Read the model definition and answer for the solid it produces. Units are mm, in the model's axes. Face numbers are marked on the shaded views. A direction names the side the tool comes from. Round coordinates to 2 decimals unless told otherwise and drop trailing zeros. Order: outer loops, then holes, each group sorted by start corner. A loop starts at its lowest first (then second) coordinate and runs counter-clockwise, first axis right, second up. Notation, with made-up numbers: (4, -1.75) - (16, -1.75) arc R11 ccw to (16, 4.25) - close; hole circle Ø9 at (3.25, 26.5). An arc over 180 degrees is marked (long way). Put each result on its own line as item: value. Start each with the question number.
Q1. Section D-D on x = 36.5 is taken. Give the vertices of the cut face in (y, z), then the cut area to 3 significant figures.
Q2. Each of these flat-tipped pins is pushed along its axis until it touches: pin 1 Ø3.5 at (y, z) = (-22, -43.5) entering from -X; pin 2 Ø2 at (y, z) = (-4.5, 16.5) entering from -X; pin 3 Ø1 at (y, z) = (-8.5, -27.5) entering from -X. Where does it stop, or does it pass through?
Q3. Which of the six approach directions +Z, -Z, +X, -X, +Y, -Y give full straight-line access (tool end or side, diameter ignored) to the marked faces 5, 6, 7, 8 and 9?
Q4. For a pull along X with two mould halves and no side action, classify the marked faces 1, 2, 3 and 4 as pulls with the +X half, pulls with the -X half, needs draft (parallel to the pull), parting line crosses it, or undercut.
Q5. Section C-C on y = -19.5 is taken. Give the vertices of the cut face in (x, z) (3 decimals).
Q6. Section A-A on x = 20 is taken. Give the vertices of the cut face in (y, z), then the cut area to 3 significant figures.
Q7. Find the intervals of material crossed by line 1 along Z through (x, y) = (-2, -20.25); line 2 along Z through (x, y) = (49, -11.5); line 3 along Z through (x, y) = (-1, -26), in increasing order. Write a range as from..to.
Q8. Section B-B on z = -23.5 is taken. Give the vertices of the cut face in (x, y), then the cut area to 3 significant figures.
from build123d import *

# Parameters (mm, degrees)
F0_W      = 71.12
F0_H      = 28.448
F1_DEPTH  = 28.448
F3_DEPTH  = 25.4
F4_DEPTH  = 25.4
F6_DEPTH  = 29.3733245078
F8_DEPTH  = 29.3562148671
F9_W      = 26.5992027439
F9_H      = 25.4
F10_DEPTH = 29.3562148671
F12_DEPTH = 50.8
F14_DEPTH = 25.3715035059
F16_DEPTH = 29.4182237139
F18_DEPTH = 29.4182237139


with BuildPart() as f1:
    # F0 (on Front) → F1 (new body)
    with BuildSketch(Plane.XZ):
        with Locations((4.2755420916, -14.224)):
            Rectangle(F0_W, F0_H)
    extrude(amount=F1_DEPTH)

    # F2 (on face) → F3 (join)
    with BuildSketch(Plane.XY):
        Polygon((39.8355420916, -6.35), (-31.2844579084, -6.35), (-31.2844579084, -21.59), (-24.3643354625, -21.59), (-24.3643354625, -26.416), (39.8355420916, -26.416), align=None)
        Polygon((39.8355420916, 0), (39.8355420916, -6.35), (39.8355420916, -26.416), (39.8355420916, -28.448), (66.4746039532, -29.3723245078), (66.4906352758, 0), align=None)
    extrude(amount=-F3_DEPTH)

    # F2 (on face) → F4 (join)
    with BuildSketch(Plane.XY):
        Polygon((39.8355420916, -6.35), (-31.2844579084, -6.35), (-31.2844579084, -21.59), (-24.3643354625, -21.59), (-24.3643354625, -26.416), (39.8355420916, -26.416), (39.8355420916, -28.448), (66.4746039532, -29.3723245078), (66.4906352758, 0), (39.8355420916, 0), align=None)
    extrude(amount=F4_DEPTH)

    # F5 (on Front) → F6 (cut, through all)
    with BuildSketch(Plane.XZ):
        with BuildLine():
            Line((13.9288037957, 18.2963101068), (-12.0401520726, 18.2963101068))
            ThreePointArc((-12.0401520726, 18.2963101068), (-16.6437398491, 13.6927223303), (-12.0401520726, 9.0891345539))
            Line((-12.0401520726, 9.0891345539), (13.9288037957, 9.0891345539))
            ThreePointArc((13.9288037957, 9.0891345539), (18.5323915722, 13.6927223303), (13.9288037957, 18.2963101068))
        make_face()
        Polygon((69.9178975219, 28.448), (39.8913989174, 0), (69.9178975219, 0), align=None)
    extrude(amount=F6_DEPTH, mode=Mode.SUBTRACT)

    # F7 (on face) → F8 (cut, through all)
    with BuildSketch(Plane(origin=(-0.9380015967, -27.0332360006, 0), x_dir=(0.9993985644, -0.0346772191, 0), z_dir=(-0.0346772191, -0.9993985644, 0))):
        Polygon((54.266725333, 12.7), (40.7980811078, 12.7), (40.8539715481, 0), align=None)
    extrude(amount=-F8_DEPTH, mode=Mode.SUBTRACT)

    # F9 (on face) → F10 (cut, through all)
    with BuildSketch(Plane(origin=(-0.9380015967, -27.0332360006, 0), x_dir=(0.9993985644, -0.0346772191, 0), z_dir=(-0.0346772191, -0.9993985644, 0))):
        with Locations((54.15357292, -12.7)):
            Rectangle(F9_W, F9_H)
    extrude(amount=-F10_DEPTH, mode=Mode.SUBTRACT)

    # F11 (on Top) → F12 (join)
    with BuildSketch(Plane.XY):
        Polygon((39.5289533985, -6.35), (-31.5910466015, -6.35), (-31.0273190044, -20.828), (-20.2347878367, -20.828), (-20.2347878367, -25.3705035059), (33.4493406117, -25.3705035059), (39.5289533985, -25.3705035059), (39.5289533985, -28.8873665619), (65.7633790028, -29.4085801184), (65.7633790028, 0), (39.5289533985, 0), align=None)
    extrude(amount=-F12_DEPTH)

    # F13 (on face) → F14 (cut, through all)
    with BuildSketch(Plane.XZ.offset(25.3705035059)):
        with BuildLine():
            Line((18.4132819485, -33.5730523437), (-10.3250071326, -33.5730523437))
            ThreePointArc((-10.3250071326, -33.5730523437), (-14.1350071326, -37.3830523437), (-10.3250071326, -41.1930523437))
            Line((-10.3250071326, -41.1930523437), (18.4132819485, -41.1930523437))
            ThreePointArc((18.4132819485, -41.1930523437), (22.4639207193, -37.3830523437), (18.4132819485, -33.5730523437))
        make_face()
    extrude(amount=-F14_DEPTH, mode=Mode.SUBTRACT)

    # F15 (on face) → F16 (cut, through all)
    with BuildSketch(Plane(origin=(-0.5580978428, -28.0909353817, 0), x_dir=(0.9998026988, -0.0198636223, 0), z_dir=(-0.0198636223, -0.9998026988, 0))):
        Polygon((66.3345647354, 0), (40.0949620257, 0), (40.0949620257, -29.1759762913), (66.3345647354, -50.8), align=None)
    extrude(amount=-F16_DEPTH, mode=Mode.SUBTRACT)

    # F17 (on face) → F18 (cut, through all)
    with BuildSketch(Plane(origin=(-0.5580978428, -28.0909353817, 0), x_dir=(0.9998026988, -0.0198636223, 0), z_dir=(-0.0198636223, -0.9998026988, 0))):
        Polygon((50.5786476823, -37.8155685024), (40.0949620257, -29.1759762913), (40.0949620257, -37.8155685024), align=None)
    extrude(amount=-F18_DEPTH, mode=Mode.SUBTRACT)


solid = f1.part
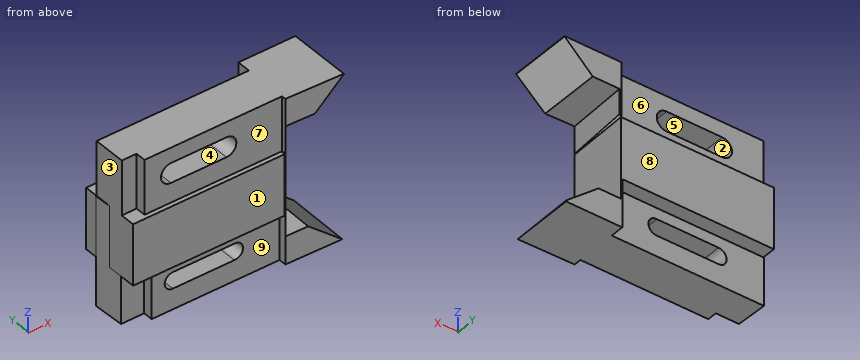
Findings:
1. outline: (-28.45, -28.45) - (-25.37, -28.45) - (-25.37, -50.8) - (-6.35, -50.8) - (-6.35, -28.45) - (0, -28.45) - (0, 0) - (-6.35, 0) - (-6.35, 25.4) - (-26.42, 25.4) - (-26.42, 0) - (-28.45, 0) - close
1. area: 1,740 mm2
2. pin 1: x = -31.05
2. pin 2: x = 39.84
2. pin 3: x = -31.53
3. face 5: +Y, -Y
3. face 6: +Z, -X, +Y
3. face 7: +Z, -X, -Y
3. face 8: +Z, -Z, +X, -X, +Y
3. face 9: -Z, -X, -Y
4. face 1: needs draft
4. face 2: undercut
4. face 3: pulls with the -X half
4. face 4: undercut
5. outline: (-31.284, -28.448) - (-31.079, -28.448) - (-31.079, -50.8) - (65.763, -50.8) - (65.763, -50.638) - (50.201, -37.816) - (39.715, -37.816) - (39.715, 0) - (39.891, 0) - (40.201, 0.293) - (40.146, 12.7) - (53.296, 12.7) - (66.48, 25.191) - (66.48, 25.4) - (-31.284, 25.4) - close; hole (-12.04, 9.089) - (13.929, 9.089) arc R4.604 ccw to (13.929, 18.296) - (-12.04, 18.296) arc R4.604 ccw to start; hole (-10.325, -41.193) - (18.413, -41.193) arc R3.817 ccw (long way) to (18.413, -33.573) - (-10.325, -33.573) arc R3.81 ccw to start
6. outline: (-28.45, -28.45) - (-25.37, -28.45) - (-25.37, -33.81) - (-6.35, -33.81) - (-6.35, -28.45) - (0, -28.45) - (0, 0) - (-6.35, 0) - (-6.35, 25.4) - (-26.42, 25.4) - (-26.42, 0) - (-28.45, 0) - close; (-25.37, -50.8) - (-6.35, -50.8) - (-6.35, -40.95) - (-25.37, -40.95) - close
6. area: 1,610 mm2
7. line 1: -50.8..-41.19, -33.57..9.09, 18.3..25.4
7. line 2: -50.8..-37.82, 12.7..25.4
7. line 3: -28.45..9.09, 18.3..25.4
8. outline: (-31.59, -6.35) - (-31.28, -14.22) - (-31.28, -28.45) - (39.53, -28.45) - (39.53, -28.89) - (40.1, 0) - (-31.28, 0) - (-31.28, -6.35) - close
8. area: 2,020 mm2
